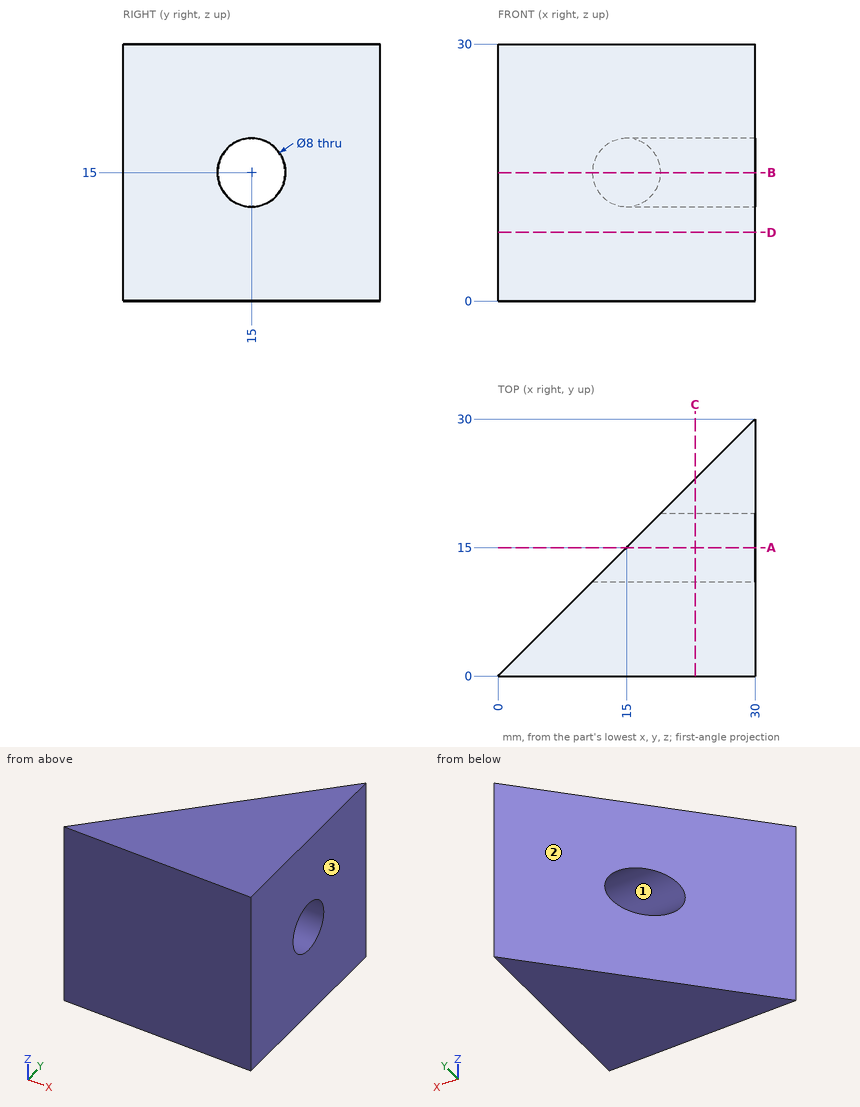
Verification items for this drawing (mm, ordinates from the low corner). Give positions to 0.01 mm unless a question says otherwise; leave off trailing zeros. Loops run counter-clockwise (first coordinate to the right, second up) from the corner with the lowest first, then second, coordinate; pieces in that order, holes last. Notation, with made-up numbers: M 38,62.5 L 97,62.5 A15 ccw 97,79.5 Z; hole C 68.25,-20.75 d9. An arc over 180 degrees is marked long. Return JSON: item names as keys, results as strings. Group by question number.
1. Mould release check, pull along X, two halves, no side actions. Record for the marked faces 1, 2 and 3: released by +X, released by -X, zero draft, split by the parting line, or undercut.
2. Cross-section at A-A on y = 15. Record the boundary of the cut face in (x, z).
3. Cross-section at B-B on z = 15. Record the boundary of the cut face in (x, y).
4. Go/stop test with flat-tipped pins: pin 1 (5 mm diameter, centred on x = 23.5, z = 24, fed in from -Y); pin 2 (2 mm diameter, centred on x = 26, z = 13, fed in from +Y); pin 3 (4 mm diameter, centred on y = 16, z = 23.5, fed in from -X); pin 4 (1 mm diameter, centred on y = 4, z = 13.5, fed in from -X). Record where each tip stops, or that it passes through.
5. Cross-section at D-D on z = 8. Record the boundary of the cut face in (x, y).
6. Thickness scan on L1, parallel to Z at x = 20.75, y = 15; L2, parallel to Y at x = 19, z = 2; L3, parallel to Y at x = 21.5, z = 16. Record the ranges inside material, lowest first.
7. Cross-section at C-C on x = 23. Record the boundary of the cut face in (y, z), plus the area to 3 significant figures.
Return value:
{
 "1": {"face 1": "zero draft", "face 2": "released by -X", "face 3": "released by +X"},
 "2": {"outline": "M 15,0 L 30,0 L 30,11 L 15,11 Z; M 15,19 L 30,19 L 30,30 L 15,30 Z"},
 "3": {"outline": "M 0,0 L 30,0 L 30,11 L 11,11 Z; M 19,19 L 30,19 L 30,30 Z"},
 "4": {"pin 1": "y = 0", "pin 2": "y = 27", "pin 3": "x = 14", "pin 4": "x = 3.5"},
 "5": {"outline": "M 0,0 L 30,0 L 30,30 Z"},
 "6": {"L1": "0 to 11, 19 to 30", "L2": "0 to 19", "L3": "0 to 11.13, 18.87 to 21.5"},
 "7": {"outline": "M 0,0 L 23,0 L 23,30 L 0,30 Z; hole C 15,15 d8", "area": "640 mm^2"}
}
